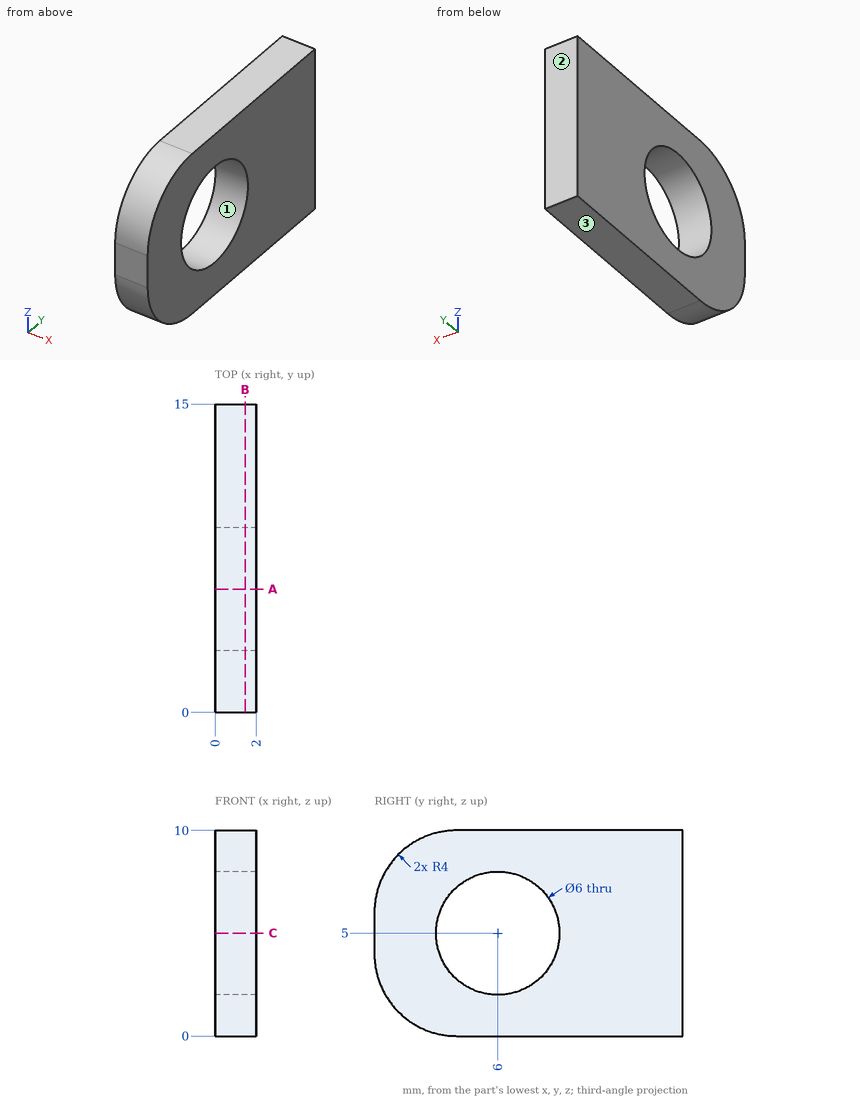
Check sheet for the drawn part. Datum: minimum x, y, z corner. Units: mm. Round coordinates to 2 decimals unless told otherwise and drop trailing zeros. Write each loop counter-clockwise with the first axis right and the second up, starting at its lowest first coordinate (ties: lowest second). Pieces come first, ordered by that corner, then holes. Notation, with made-up numbers: (78.25, 34.25) -> (108.25, 34.25) arc R20 cw to (108.25, 38.25) -> close; hole circle Ø1 at (-36.5, -39.75). An arc over 180 degrees is marked (long way). Put each result on its own line as item: value.
(1) Sectioned sample at B-B (x = 1.45). Enter the section's corners in (y, z), plus the area to 3 significant figures.
Values found:
outline: (0, 4) arc R4 ccw to (4, 0) -> (15, 0) -> (15, 10) -> (4, 10) arc R4 ccw to (0, 6) -> close; hole circle Ø6 at (6, 5)
area: 115 mm^2
(2) Go/stop test with a flat-tipped pin: pin 1 Ø6 at (y, z) = (7.5, 8.5) entering from -X. Record where the tip stops, or that it passes through.
Values found:
pin 1: stops at x = 0
(3) Mould release check, pull along Y, two halves, no side actions. Record for the marked faces 1, 2 and 3: released by +Y, released by -Y, zero draft, split by the parting line, or undercut.
Values found:
face 1: undercut
face 2: released by +Y
face 3: zero draft
(4) Material ranges on line 1 (Y direction, x = 0.7, z = 5); line 2 (Z direction, x = 1.35, y = 6); line 3 (Y direction, x = 0.55, z = 2.5), recorded low to high.
Values found:
line 1: y = 0 to 3, 9 to 15
line 2: z = 0 to 2, 8 to 10
line 3: y = 0.29 to 4.34, 7.66 to 15
(5) Sectioned sample at C-C (z = 5). Enter the section's corners in (x, y), plus the area to 3 significant figures.
Values found:
outline: (0, 0) -> (2, 0) -> (2, 3) -> (0, 3) -> close; (0, 9) -> (2, 9) -> (2, 15) -> (0, 15) -> close
area: 18.0 mm^2
(6) Sectioned sample at A-A (y = 6). Enter the section's corners in (x, z), plus the area to 3 significant figures.
Values found:
outline: (0, 0) -> (2, 0) -> (2, 2) -> (0, 2) -> close; (0, 8) -> (2, 8) -> (2, 10) -> (0, 10) -> close
area: 8.00 mm^2
